Read the model definition and answer for the solid it produces. Units are mm, in the model's axes. A direction names the side the tool comes from. Coordinates: 2 decimals unless noted, no trailing zeros. Write each loop counter-clockwise with the first axis right and the second up, starting at its lowest first coordinate (ties: lowest second). Pieces come first, ordered by that corner, then holes. Notation, with made-up numbers: (-16, 14) -> (35, 14) arc R17 ccw to (35, 37) -> close; hole circle Ø3 at (30, 47.25). An arc over 180 degrees is marked (long way). Answer as a JSON object with one key per item and string values. Group by question number.
(1) For a pull along Y with two mould halves and no side action, classify faces 4 (the face through (19, 55, 38)), 5 (the face through (-17.84, 17.42, 51.29)), 6 (the face through (-36, 73.57, 87.32)), 7 (the face through (0, 38, 73)) as +Y half, -Y half, draft (parallel to the pull), parting line (faces both ways), or undercut.
(2) Straight lines are drawn through the part: L1, parallel to X at y = 38, z = 82.5; L2, parallel to Y at x = 0, z = 82; L3, parallel to X at y = 54.5, z = 74.5. For each, find the intervals that lie inside material, in ascending order.
(3) Flat-ended cylindrical pins translate along their axes: P1, Ø0.6, axis at y = 75.5, z = 71, coming from the -X side; P2, Ø1, axis at x = -6.5, y = 76.5, coming from the +Z side; P3, Ø4, axis at x = -15.5, y = 34, coming from the +Z side. Find the tip coordinate at first contact, or state that the pin passes through.
(4) Which of the six approach directions +Z, -Z, +X, -X, +Y, -Y give full straight-line access (tool end or side, diameter ignored) to faces 1 (the face through (-7.1, 5.53, 86.69)), 2 (the face through (0, 75, 80)), 3 (the face through (-1, 74, 98))?
(5) Find section B-B (y = 54.5). Give the vertices of the cut face in (x, z), then the cut area to 3 significant figures.
(6) Find section A-A (y = 23). Give the vertices of the cut face in (x, z), then the cut area to 3 significant figures.
from build123d import *

# Parameters (mm, degrees)
CROQUIS1_W              = 37.5
CROQUIS1_H              = 25
SALIENTE_EXTRUIR1_DEPTH = 75
CROQUIS3_R              = 32.75
CORTAR_EXTRUIR2_DEPTH   = 27
REDONDEO4_R             = 40
REDONDEO5_R             = 5
CROQUIS4_W              = 30
CROQUIS4_H              = 30
SALIENTE_EXTRUIR2_DEPTH = 2
CROQUIS5_W              = 8
CROQUIS5_H              = 8
CORTAR_EXTRUIR10_DEPTH  = 2


with BuildPart() as part:
    # Croquis1 → Saliente-Extruir1 (new body)
    with BuildSketch(Plane(origin=(0, 0, 0), x_dir=(1, 0, 0), z_dir=(0, 1, 0))):
        Polygon((0, 0), (-37.5, -75), (0, -75), align=None)
        Polygon((37.5, -75), (0, 0), (0, -75), align=None)
        with Locations((18.75, -87.5)):
            Rectangle(CROQUIS1_W, CROQUIS1_H)
        with Locations((-18.75, -87.5)):
            Rectangle(CROQUIS1_W, CROQUIS1_H)
    extrude(amount=SALIENTE_EXTRUIR1_DEPTH)

    # Croquis3 → Cortar-Extruir2 (cut)
    with BuildSketch(Plane.XY.offset(100)):
        with Locations((0, 37.5)):
            Circle(CROQUIS3_R)
    extrude(amount=-CORTAR_EXTRUIR2_DEPTH, mode=Mode.SUBTRACT)

    # Redondeo4
    redondeo4_edges = [part.edges().sort_by_distance(p)[0] for p in [
        (-18.75, 0, 37.5),
        (18.75, 0, 37.5),
    ]]
    fillet(redondeo4_edges, radius=REDONDEO4_R)

    # Redondeo5
    # the kernel refuses this fillet: 5 mm, written as the material it takes off along each edge
    with BuildSketch(Plane(origin=(37.5, 75, 112.5), x_dir=(-1, 0, 0), z_dir=(0, 0, -1)), Plane(origin=(-37.5, 75, 62.5), x_dir=(1, 0, 0), z_dir=(0, 0, 1))) as redondeo5_piece_1:
        with BuildLine():
            CenterArc((REDONDEO5_R, -REDONDEO5_R), REDONDEO5_R, 90, 90)
            Line((0, -REDONDEO5_R), (0, 0))
            Line((0, 0), (REDONDEO5_R, 0))
        make_face()
    extrude(amount=50, mode=Mode.SUBTRACT)
    with BuildSketch(Plane(origin=(43.090169944, 75, 86.180339887), x_dir=(0, -1, 0), z_dir=(-0.4472135954999581, 0, -0.8944271909999159)), Plane(origin=(5.590169944, 75, -11.180339887), x_dir=(0, -1, 0), z_dir=(-0.44721359549995776, 0, 0.894427190999916))) as redondeo5_piece_2:
        with BuildLine():
            CenterArc((REDONDEO5_R, REDONDEO5_R), REDONDEO5_R, 180, 90)
            Line((0, REDONDEO5_R), (0, 0))
            Line((0, 0), (REDONDEO5_R, 0))
        make_face()
    extrude(amount=108.852549156, mode=Mode.SUBTRACT)
    with BuildSketch(Plane(origin=(-50, 75, 100), x_dir=(0, 0, -1), z_dir=(1, 0, 0))) as redondeo5_piece_3:
        with BuildLine():
            CenterArc((REDONDEO5_R, -REDONDEO5_R), REDONDEO5_R, 90, 90)
            Line((0, -REDONDEO5_R), (0, 0))
            Line((0, 0), (REDONDEO5_R, 0))
        make_face()
    extrude(amount=100, mode=Mode.SUBTRACT)

    # Croquis4 → Saliente-Extruir2 (add)
    with BuildSketch(Plane(origin=(0, 75, 0), x_dir=(1, 0, 0), z_dir=(0, 1, 0))):
        with Locations((0, -80)):
            Rectangle(CROQUIS4_W, CROQUIS4_H)
    extrude(amount=SALIENTE_EXTRUIR2_DEPTH)

    # Croquis5 → Cortar-Extruir10 (cut)
    with BuildSketch(Plane(origin=(0, 77, 0), x_dir=(1, 0, 0), z_dir=(0, 1, 0))):
        with Locations((-8.012274888, -88.012274888)):
            Rectangle(CROQUIS5_W, CROQUIS5_H)
        with Locations((8.001867248, -71.998132752)):
            Rectangle(CROQUIS5_W, CROQUIS5_H)
        with Locations((-0.00520382, -80.00520382)):
            Rectangle(CROQUIS5_W, CROQUIS5_H)
    extrude(amount=-CORTAR_EXTRUIR10_DEPTH, mode=Mode.SUBTRACT)


solid = part.part
Results below:
{
 "1": {"face 4": "draft", "face 5": "-Y half", "face 6": "+Y half", "face 7": "undercut"},
 "2": {"L1": "x = -37.5 to -32.75, 32.75 to 37.5", "L2": "y = 0.14 to 4.75, 70.25 to 75", "L3": "x = -37.25 to -27.99, 27.99 to 37.25"},
 "3": {"P1": "stops at x = -15", "P2": "stops at z = 95", "P3": "stops at z = 73"},
 "4": {"face 1": "+Z", "face 2": "+Y", "face 3": "+Z, +X, -X, +Y"},
 "5": {"outline": "(-37.5, 75) -> (0, 0) -> (37.5, 75) -> (37.5, 100) -> (27.99, 100) -> (27.99, 73) -> (-27.99, 73) -> (-27.99, 100) -> (-37.5, 100) -> close", "area": "3,180 mm2"},
 "6": {"outline": "(-37.5, 83.48) -> (0, 8.48) -> (37.5, 83.48) -> (37.5, 100) -> (29.37, 100) -> (29.37, 73) -> (-29.37, 73) -> (-29.37, 100) -> (-37.5, 100) -> close", "area": "2,470 mm2"}
}
